Build history of the part. All positions in model axes, mm. Round coordinates to 2 decimals unless told otherwise and drop trailing zeros. Order: outer loops, then holes, each group sorted by start corner. A loop starts at its lowest first (then second) coordinate and runs counter-clockwise, first axis right, second up. Notation, with made-up numbers: (10, -24) -> (36, -24) arc R12 cw to (36, -11) -> close; hole circle Ø2 at (50.5, -15.5). An arc over 180 degrees is marked (long way). Use a Markdown table: item, result. Add a question column.
Item 1: Slice it at A-A, the plane x = 0. Give the cut face in (y, z), plus the area to 3 significant figures.
Item 2: Probe L1, parallel to X at y = 17.5, z = 28; L2, parallel to X at y = 15.5, z = 10; L3, parallel to Y at x = 21, z = 18. List the from-to ranges inside material, lowest first.
Item 3: Slice it at B-B, the plane y = 0. Give the cut face in (x, z).
Item 4: Slice it at D-D, the plane z = 36.5. Give the cut face in (x, y), plus the area to 3 significant figures.
Item 5: Pin check, flat tips, straight feed: pin 1 (4 mm diameter, centred on y = -10, z = 35, fed in from -X); pin 2 (2 mm diameter, centred on x = 17, z = 19.5, fed in from +Y); pin 3 (1.5 mm diameter, centred on x = 9, z = 15, fed in from -Y); pin 4 (10 mm diameter, centred on x = 16, y = 16.5, fed in from -Z). Stop position of each tip, or through.
Item 6: Slice it at C-C, the plane y = -11.5. Give the cut face in (x, z), plus the area to 3 significant figures.
Item 7: Two-plate mould, pull along X, no slides. Class faces 1 (the face through (11.2, 6.1, 0)), 2 (the face through (-20.633, -15.821, 19.72)), 3 (the face through (11.733, -16.563, 19.72)): released by +X, released by -X, zero draft, split by the parting line, or undercut.
from build123d import *

# Parameters (mm, degrees)
SKETCH_1_R          = 26
SKETCH_1_R_2        = 2.25
EXTRUDE_1_DEPTH     = 40
SKETCH_2_R          = 12.5
CUT_EXTRUDE_1_DEPTH = 55.332310829


with BuildPart() as part:
    # 草图1 → 凸台-拉伸1 (new body)
    with BuildSketch(Plane.XY):
        Circle(SKETCH_1_R)
        with Locations((-21.75, 0)):
            Circle(SKETCH_1_R_2, mode=Mode.SUBTRACT)
        with Locations((-13.980630511, 16.661466638)):
            Circle(SKETCH_1_R_2, mode=Mode.SUBTRACT)
        with Locations((-13.980630511, -16.661466638)):
            Circle(SKETCH_1_R_2, mode=Mode.SUBTRACT)
        with Locations((13.980630511, -16.661466638)):
            Circle(SKETCH_1_R_2, mode=Mode.SUBTRACT)
        with Locations((21.75, 0)):
            Circle(SKETCH_1_R_2, mode=Mode.SUBTRACT)
        with Locations((13.980630511, 16.661466638)):
            Circle(SKETCH_1_R_2, mode=Mode.SUBTRACT)
    extrude(amount=EXTRUDE_1_DEPTH)

    # 草图2 → 切除-拉伸1 (cut, through all)
    with BuildSketch(Plane.XY.offset(40)):
        Circle(SKETCH_2_R)
    extrude(amount=-CUT_EXTRUDE_1_DEPTH, mode=Mode.SUBTRACT)


solid = part.part
Check sheet entries:
| question | item | result |
|---|---|---|
| 1 | outline | (-26, 0) -> (-12.5, 0) -> (-12.5, 40) -> (-26, 40) -> close; (12.5, 0) -> (26, 0) -> (26, 40) -> (12.5, 40) -> close |
| 1 | area | 1,080 mm2 |
| 2 | L1 | -19.23 to -16.07, -11.89 to 11.89, 16.07 to 19.23 |
| 2 | L2 | -20.87 to -15.91, -12.05 to 12.05, 15.91 to 20.87 |
| 2 | L3 | -15.33 to -2.12, 2.12 to 15.33 |
| 3 | outline | (-26, 0) -> (-24, 0) -> (-24, 40) -> (-26, 40) -> close; (-19.5, 0) -> (-12.5, 0) -> (-12.5, 40) -> (-19.5, 40) -> close; (12.5, 0) -> (19.5, 0) -> (19.5, 40) -> (12.5, 40) -> close; (24, 0) -> (26, 0) -> (26, 40) -> (24, 40) -> close |
| 4 | outline | circle Ø52 at (0, 0); hole circle Ø4.5 at (-21.75, 0); hole circle Ø4.5 at (-13.98, -16.66); hole circle Ø4.5 at (-13.98, 16.66); hole circle Ø25 at (0, 0); hole circle Ø4.5 at (13.98, -16.66); hole circle Ø4.5 at (13.98, 16.66); hole circle Ø4.5 at (21.75, 0) |
| 4 | area | 1,540 mm2 |
| 5 | pin 1 | x = -24.74 |
| 5 | pin 2 | y = 20.49 |
| 5 | pin 3 | y = -24.66 |
| 5 | pin 4 | z = 0 |
| 6 | outline | (-23.32, 0) -> (-4.9, 0) -> (-4.9, 40) -> (-23.32, 40) -> close; (4.9, 0) -> (23.32, 0) -> (23.32, 40) -> (4.9, 40) -> close |
| 6 | area | 1,470 mm2 |
| 7 | face 1 | zero draft |
| 7 | face 2 | split by the parting line |
| 7 | face 3 | undercut |
